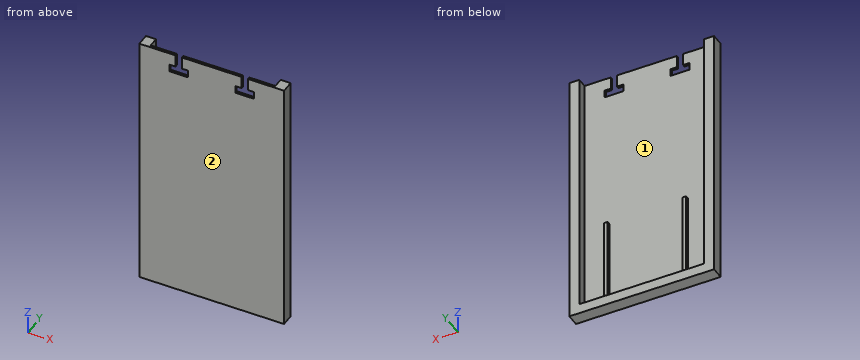
```python
from build123d import *

# Parameters (mm, degrees)
SKETCH3_W               = 116
SKETCH3_H               = 416
BOSS_EXTRUDE1_DEPTH     = 10
SKETCH4_W               = 100
SKETCH4_H               = 400
CUT_EXTRUDE1_DEPTH      = 8
SKETCH6_W               = 3
SKETCH6_H               = 100
BOSS_EXTRUDE4_DEPTH     = 3
SKETCH7_R               = 1.5
BOSS_EXTRUDE5_DEPTH     = 3
CUT_EXTRUDE2_DEPTH      = 10
CUT_EXTRUDE2_DEPTH_BACK = 10
SKETCH8_W               = 116
SKETCH8_H               = 176.78031556
CUT_EXTRUDE4_DEPTH      = 37
CUT_EXTRUDE5_DEPTH      = 10
SKETCH11_W              = 8
SKETCH11_H              = 30
CUT_EXTRUDE6_DEPTH      = 10
SKETCH12_W              = 3
SKETCH12_H              = 30
CUT_EXTRUDE7_DEPTH      = 10
SKETCH13_W              = 3
SKETCH13_H              = 30
CUT_EXTRUDE10_DEPTH     = 14
SKETCH14_W              = 3
SKETCH14_H              = 30
BOSS_EXTRUDE8_DEPTH     = 2


with BuildPart() as part:
    # Sketch3 → Boss-Extrude1 (new body)
    with BuildSketch(Plane(origin=(0, 0, 0), x_dir=(1, 0, 0), z_dir=(0, 1, 0))):
        with Locations((-1098.104867157, 569.267379684)):
            Rectangle(SKETCH3_W, SKETCH3_H)
    extrude(amount=BOSS_EXTRUDE1_DEPTH)

    # Sketch4 → Cut-Extrude1 (cut)
    with BuildSketch(Plane(origin=(0, 10, 0), x_dir=(1, 0, 0), z_dir=(0, 1, 0))):
        with Locations((-1098.104867157, 569.267379684)):
            Rectangle(SKETCH4_W, SKETCH4_H)
    extrude(amount=-CUT_EXTRUDE1_DEPTH, mode=Mode.SUBTRACT)

    # Sketch6 → Boss-Extrude4 (add)
    with BuildSketch(Plane(origin=(0, 2, 0), x_dir=(1, 0, 0), z_dir=(0, 1, 0))):
        with Locations((-1129.604867157, 719.267379684)):
            Rectangle(SKETCH6_W, SKETCH6_H)
        with Locations((-1066.604867157, 719.267379684)):
            Rectangle(SKETCH6_W, SKETCH6_H)
    extrude(amount=BOSS_EXTRUDE4_DEPTH)

    # Sketch7 → Boss-Extrude5 (add)
    with BuildSketch(Plane(origin=(0, 2, 0), x_dir=(1, 0, 0), z_dir=(0, 1, 0))):
        with Locations(Location((-1085.404867157, 452.168271652, 0), (0, 0, 270))):
            Circle(SKETCH7_R)
    extrude(amount=BOSS_EXTRUDE5_DEPTH)

    # Sketch8 → Cut-Extrude2 (cut, two sides: drawn at the far end of the back side and taken through both)
    with BuildSketch(Plane(origin=(0, 2, 0), x_dir=(1, 0, 0), z_dir=(0, 1, 0)).offset(-CUT_EXTRUDE2_DEPTH_BACK)):
        with Locations((-1098.104867157, 449.657537464)):
            Rectangle(SKETCH8_W, SKETCH8_H)
    extrude(amount=CUT_EXTRUDE2_DEPTH + CUT_EXTRUDE2_DEPTH_BACK, mode=Mode.SUBTRACT)

    # Sketch9 → Cut-Extrude4 (cut)
    with BuildSketch(Plane(origin=(0, 2, 0), x_dir=(1, 0, 0), z_dir=(0, 1, 0))):
        Polygon((-1127.104867157, 548.047695244), (-1127.104867157, 538.047695244), (-1122.104867157, 538.047695244), (-1122.104867157, 548.047695244), (-1117.104867157, 548.047695244), (-1117.104867157, 554.047695244), (-1132.104867157, 554.047695244), (-1132.104867157, 548.047695244), align=None)
        Polygon((-1074.104867157, 548.047695244), (-1074.104867157, 538.047695244), (-1069.104867157, 538.047695244), (-1069.104867157, 548.047695244), (-1064.104867157, 548.047695244), (-1064.104867157, 554.047695244), (-1079.104867157, 554.047695244), (-1079.104867157, 548.047695244), align=None)
    extrude(amount=-CUT_EXTRUDE4_DEPTH, mode=Mode.SUBTRACT)

    # Sketch10 → Cut-Extrude5 (cut)
    with BuildSketch(Plane(origin=(0, 5, 0), x_dir=(1, 0, 0), z_dir=(0, 1, 0))):
        Polygon((-1127.104867157, 578.047695244), (-1127.104867157, 568.047695244), (-1122.104867157, 568.047695244), (-1122.104867157, 578.047695244), (-1117.104867157, 578.047695244), (-1117.104867157, 584.047695244), (-1132.104867157, 584.047695244), (-1132.104867157, 578.047695244), align=None)
        Polygon((-1156.104867157, 568.047695244), (-1156.104867157, 538.047695244), (-1040.104867157, 538.047695244), (-1040.104867157, 568.047695244), (-1069.104867157, 568.047695244), (-1074.104867157, 568.047695244), (-1122.104867157, 568.047695244), (-1127.104867157, 568.047695244), align=None)
        Polygon((-1069.104867157, 568.047695244), (-1074.104867157, 568.047695244), (-1074.104867157, 578.047695244), (-1079.104867157, 578.047695244), (-1079.104867157, 584.047695244), (-1064.104867157, 584.047695244), (-1064.104867157, 578.047695244), (-1069.104867157, 578.047695244), align=None)
    extrude(amount=-CUT_EXTRUDE5_DEPTH, mode=Mode.SUBTRACT)

    # Sketch11 → Cut-Extrude6 (cut)
    with BuildSketch(Plane(origin=(0, 0, 0), x_dir=(1, 0, 0), z_dir=(0, 1, 0))):
        with Locations((-1152.104867157, 553.047695244)):
            Rectangle(SKETCH11_W, SKETCH11_H)
        with Locations((-1044.104867157, 553.047695244)):
            Rectangle(SKETCH11_W, SKETCH11_H)
    extrude(amount=CUT_EXTRUDE6_DEPTH, mode=Mode.SUBTRACT)

    # Sketch12 → Cut-Extrude7 (cut)
    with BuildSketch(Plane(origin=(0, 2, 0), x_dir=(1, 0, 0), z_dir=(0, 1, 0))):
        with Locations((-1066.604867157, 684.267379684)):
            Rectangle(SKETCH12_W, SKETCH12_H)
    extrude(amount=CUT_EXTRUDE7_DEPTH, mode=Mode.SUBTRACT)

    # Sketch13 → Cut-Extrude10 (cut)
    with BuildSketch(Plane(origin=(0, 0, 0), x_dir=(1, 0, 0), z_dir=(0, 1, 0))):
        with Locations((-1129.604867157, 684.267379684)):
            Rectangle(SKETCH13_W, SKETCH13_H)
    extrude(amount=CUT_EXTRUDE10_DEPTH, mode=Mode.SUBTRACT)

    # Sketch14 → Boss-Extrude8 (add)
    with BuildSketch(Plane(origin=(0, 0, 0), x_dir=(1, 0, 0), z_dir=(0, 1, 0))):
        with Locations((-1129.604867157, 684.267379684)):
            Rectangle(SKETCH14_W, SKETCH14_H)
    extrude(amount=BOSS_EXTRUDE8_DEPTH)


solid = part.part
```
Build history of the part. All positions in model axes, mm. Face numbers are marked on the shaded views. Coordinates: 2 decimals unless noted, no trailing zeros. Order: outer loops, then holes, each group sorted by start corner. A loop starts at its lowest first (then second) coordinate and runs counter-clockwise, first axis right, second up. Notation, with made-up numbers: (-13, 31) -> (-2, 31) arc R18 cw to (-2, 61) -> close; hole circle Ø3 at (55, -23). An arc over 180 degrees is marked (long way). Answer in a Markdown table with one row per item. Add a question column.
Q1. Drop flat-ended pins along their axis: pin 1 (2 mm diameter, centred on x = -1129, z = -625, fed in from +Y); pin 2 (0.9 mm diameter, centred on x = -1066.5, z = -749, fed in from +Y); pin 3 (2.5 mm diameter, centred on x = -1116.5, y = 5.5, fed in from +Z). Give the stop position or say it passes through.
Q2. Band-saw the part on B-B, the plane y = 7. List the corners of the cut face in (x, z), then the cut area to 3 significant figures.
Q3. Wall check: line 1 along X through (y, z) = (3, -702.5); line 2 along X through (y, z) = (5.5, -716); line 3 along Z through (x, y) = (-1129.5, 2.5). Give the ranges that are in metal, low to high. Write a range as [from, to].
Q4. Mould opens along X. For the marked faces 1 and 2 say: +X half, -X half, draft (parallel to the pull), parting line (faces both ways), or undercut.
Q5. Band-saw the part on D-D, the plane z = -750.5. List the corners of the cut face in (x, y), then the cut area to 3 significant figures.
Q6. Band-saw the part on A-A, the plane z = -594. List the corners of the cut face in (x, y).
Q7. Band-saw the part on C-C, the plane x = -1136.5. List the corners of the cut face in (y, z).
Answers follow:
| question | item | result |
|---|---|---|
| 1 | pin 1 | y = 2 |
| 1 | pin 2 | y = 5 |
| 1 | pin 3 | z = -769.27 |
| 2 | outline | (-1156.1, -777.27) -> (-1040.1, -777.27) -> (-1040.1, -568.05) -> (-1048.1, -568.05) -> (-1048.1, -769.27) -> (-1148.1, -769.27) -> (-1148.1, -568.05) -> (-1156.1, -568.05) -> close |
| 2 | area | 4,150 mm^2 |
| 3 | line 1 | [-1156.1, -1148.1], [-1131.1, -1128.1], [-1068.1, -1065.1], [-1048.1, -1040.1] |
| 3 | line 2 | [-1156.1, -1148.1], [-1048.1, -1040.1] |
| 3 | line 3 | [-777.27, -699.27] |
| 4 | face 1 | undercut |
| 4 | face 2 | draft |
| 5 | outline | (-1156.1, 0) -> (-1040.1, 0) -> (-1040.1, 10) -> (-1048.1, 10) -> (-1048.1, 2) -> (-1065.1, 2) -> (-1065.1, 5) -> (-1068.1, 5) -> (-1068.1, 2) -> (-1128.1, 2) -> (-1128.1, 5) -> (-1131.1, 5) -> (-1131.1, 2) -> (-1148.1, 2) -> (-1148.1, 10) -> (-1156.1, 10) -> close |
| 5 | area | 378 mm^2 |
| 6 | outline | (-1156.1, 0) -> (-1040.1, 0) -> (-1040.1, 10) -> (-1048.1, 10) -> (-1048.1, 2) -> (-1148.1, 2) -> (-1148.1, 10) -> (-1156.1, 10) -> close |
| 7 | outline | (0, -777.27) -> (10, -777.27) -> (10, -769.27) -> (2, -769.27) -> (2, -568.05) -> (0, -568.05) -> close |
